Here's the drawing with two shaded views (mm, measured from the low corner). I have some questions. Round coordinates to 2 decimals unless told otherwise and drop trailing zeros. Write each loop counter-clockwise with the first axis right and the second up, starting at its lowest first coordinate (ties: lowest second). Pieces come first, ordered by that corner, then holes. Notation, with made-up numbers: M -37,-10 L -22,-10 A12 ccw -22,4 Z; hole C 45,32.5 d8. An arc over 180 degrees is marked long. Answer as a JSON object with one key per item and string values. Group by question number.
1) Please list where these lines run through material, in increasing order: L1, parallel to X at y = 1.15, z = 46; L2, parallel to X at y = 0.75, z = 25; L3, parallel to Z at x = 34, y = 0.55. Write a range as [from, to].
2) Suppose I cut it at B-B, the plane z = 25. Write out the boundary of the cut face in (x, y), and give its area (3 significant figures).
3) Suppose I cut it at C-C, the plane y = 1.05. Write out the boundary of the cut face in (x, z), and give its area (3 significant figures).
4) Suppose I cut it at A-A, the plane x = 27. Write out the boundary of the cut face in (y, z), and give its area (4 significant figures).
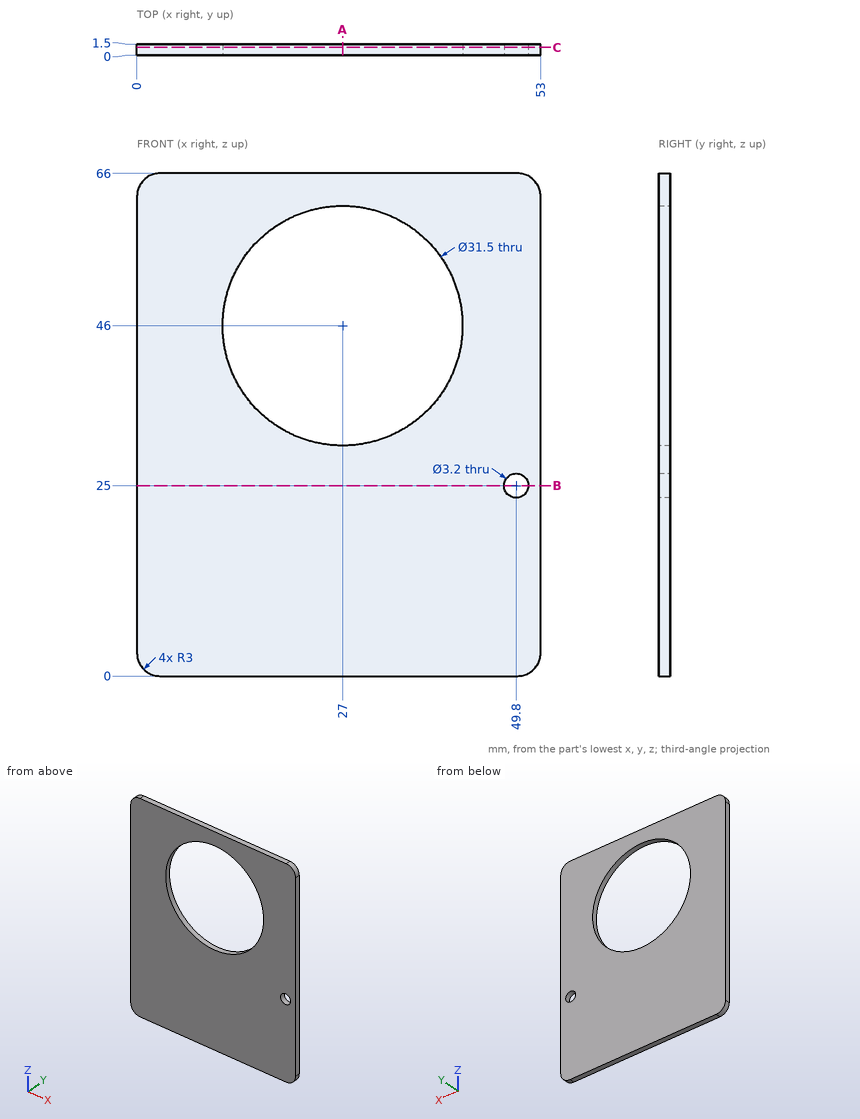
Results:
{
 "1": {"L1": "[0, 11.25], [42.75, 53]", "L2": "[0, 48.2], [51.4, 53]", "L3": "[0, 31.89], [60.11, 66]"},
 "2": {"outline": "M 0,0 L 48.2,0 L 48.2,1.5 L 0,1.5 Z; M 51.4,0 L 53,0 L 53,1.5 L 51.4,1.5 Z", "area": "74.7 mm^2"},
 "3": {"outline": "M 0,3 A3 ccw 3,0 L 50,0 A3 ccw 53,3 L 53,63 A3 ccw 50,66 L 3,66 A3 ccw 0,63 Z; hole C 27,46 d31.5; hole C 49.8,25 d3.2", "area": "2,700 mm^2"},
 "4": {"outline": "M 0,0 L 1.5,0 L 1.5,30.25 L 0,30.25 Z; M 0,61.75 L 1.5,61.75 L 1.5,66 L 0,66 Z", "area": "51.75 mm^2"}
}
